For this review, use the dimensioned drawing (mm, ordinates from the lowest corner) and the shaded views. A direction names the side the tool comes from. Give positions to 0.01 mm unless a question says otherwise; leave off trailing zeros. Write each loop counter-clockwise with the first axis right and the second up, starting at its lowest first coordinate (ties: lowest second). Pieces come first, ordered by that corner, then holes. Notation, with made-up numbers: M 27.5,66 L 46.5,66 A28 cw 46.5,99 Z; hole C 6,88.25 d8. An arc over 180 degrees is marked long. One line per item, written item: value. Start each with the question number.
Item 1: Clearance check with flat-ended pins moving along their axes: pin 1 Ø4 at (x, y) = (2.5, 15) entering from +Z; pin 2 Ø1.5 at (x, y) = (8.5, 6.5) entering from -Z. State where each tip first meets the part, or that it passes through.
Item 2: Consider section B-B, the plane y = 2.5. Write out the cut boundary in (x, z).
Item 3: Consider section D-D, the plane x = 14. Write out the cut boundary in (y, z).
Item 4: Consider section C-C, the plane z = 0.7. Write out the cut boundary in (x, y).
Item 5: Consider section A-A, the plane x = 8. Write out the cut boundary in (y, z), and give its area (3 significant figures).
Item 6: Tool access review of the marked faces 1 and 2: name each direction out of +Z, -Z, +X, -X, +Y, -Y from which nothing blocks a thin tool from reaching the whole face with its end or side.
Item 7: To check wall thickness, follow probe 1 along Z at (x, y) = (13, 12); probe 2 along X at (y, z) = (2.25, 0.1); probe 3 along Z at (x, y) = (11.5, 15.25). State the ranges of each line that lie inside material, in increasing order.
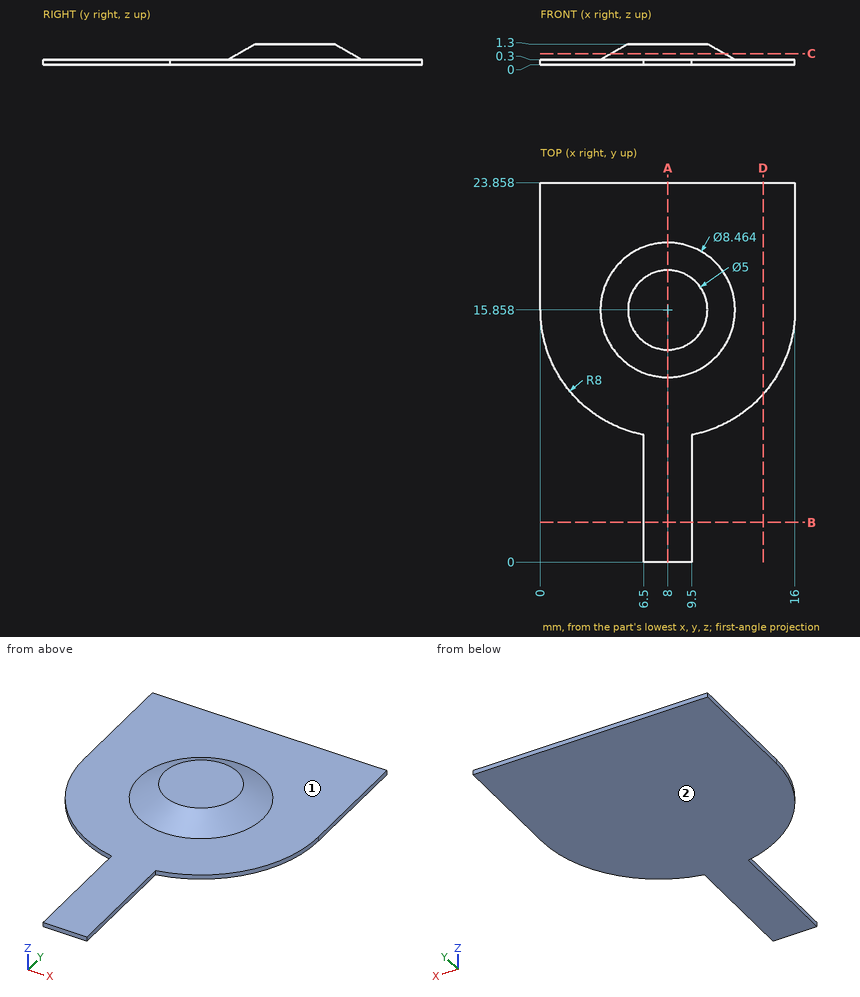
Model answer:
1. pin 1: stops at z = 0.68
1. pin 2: stops at z = 0
2. outline: M 6.5,0 L 9.5,0 L 9.5,0.3 L 6.5,0.3 Z
3. outline: M 10.57,0 L 23.86,0 L 23.86,0.3 L 10.57,0.3 Z
4. outline: C 8,15.86 d7.08
5. outline: M 0,0 L 23.86,0 L 23.86,0.3 L 20.09,0.3 L 18.36,1.3 L 13.36,1.3 L 11.63,0.3 L 0,0.3 Z
5. area: 13.9 mm2
6. face 1: +Z
6. face 2: -Z, +X, -X, +Y, -Y
7. probe 1: z = 0 to 0.3
7. probe 2: x = 6.5 to 9.5
7. probe 3: z = 0 to 0.69
